Geometry check sheet. Reference: drawing and pictorial views, mm from the part's lowest x, y, z. Round coordinates to 2 decimals unless told otherwise and drop trailing zeros. Loops run counter-clockwise (first coordinate to the right, second up) from the corner with the lowest first, then second, coordinate; pieces in that order, holes last. Notation, with made-up numbers: (-28.75, 29.5) -> (-21.75, 29.5) arc R11 cw to (-21.75, 44.5) -> close; hole circle Ø3 at (55.25, 51). An arc over 180 degrees is marked (long way). Use one line per item in the form item = value. Start each with the question number.
(1) Draft check along Y on the marked faces 1, 2 and 3. Enter one of: released by +Y, released by -Y, zero draft, split by the parting line, or undercut.
(2) Sectioned sample at C-C (z = 2.25). Record the cut outline in (x, y).
(3) Material ranges on probe 1 along Y at (x, z) = (31.75, 17.5); probe 2 along Z at (x, y) = (59, 45); probe 3 along X at (y, z) = (27, 17.25), recorded low to high. Write a range as [from, to].
(4) Go/stop test with flat-tipped pins: pin 1 (6 mm diameter, centred on y = 46.5, z = 3, fed in from +X); pin 2 (3 mm diameter, centred on x = 38, z = 15.5, fed in from +Y); pin 3 (8 mm diameter, centred on y = 53.5, z = 4.5, fed in from +X). Record where each tip stops, or that it passes through.
(5) Sectioned sample at D-D (y = 24). Record the cut outline in (x, z).
(6) Sectioned sample at A-A (x = 31.75). Record the cut outline in (y, z).
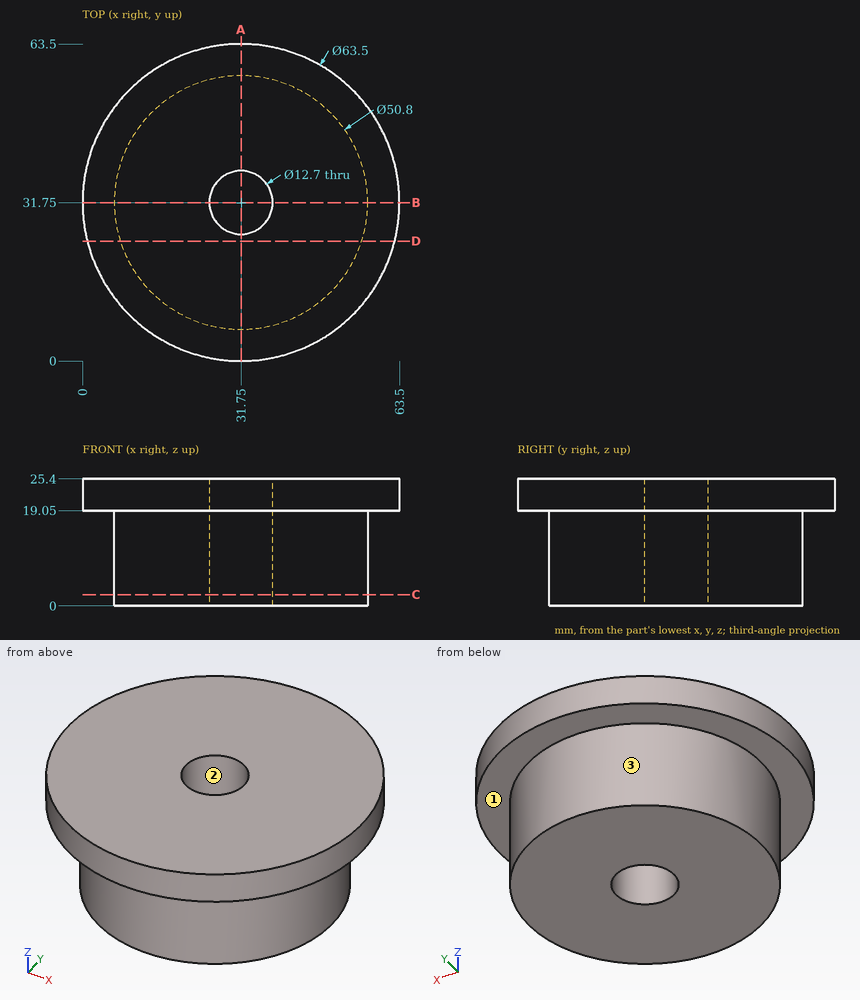
Checks:
q1.face_1 = zero draft
q1.face_2 = undercut
q1.face_3 = split by the parting line
q2.outline = circle Ø50.8 at (31.75, 31.75); hole circle Ø12.7 at (31.75, 31.75)
q3.probe_1 = [6.35, 25.4], [38.1, 57.15]
q3.probe_2 = [19.05, 25.4]
q3.probe_3 = [6.8, 27.54], [35.96, 56.7]
q4.pin_1 = 54.27
q4.pin_2 = 56.7
q4.pin_3 = 49.92
q5.outline = (0.96, 19.05) -> (7.56, 19.05) -> (7.56, 0) -> (55.94, 0) -> (55.94, 19.05) -> (62.54, 19.05) -> (62.54, 25.4) -> (0.96, 25.4) -> close
q6.outline = (0, 19.05) -> (6.35, 19.05) -> (6.35, 0) -> (25.4, 0) -> (25.4, 25.4) -> (0, 25.4) -> close; (38.1, 0) -> (57.15, 0) -> (57.15, 19.05) -> (63.5, 19.05) -> (63.5, 25.4) -> (38.1, 25.4) -> close
